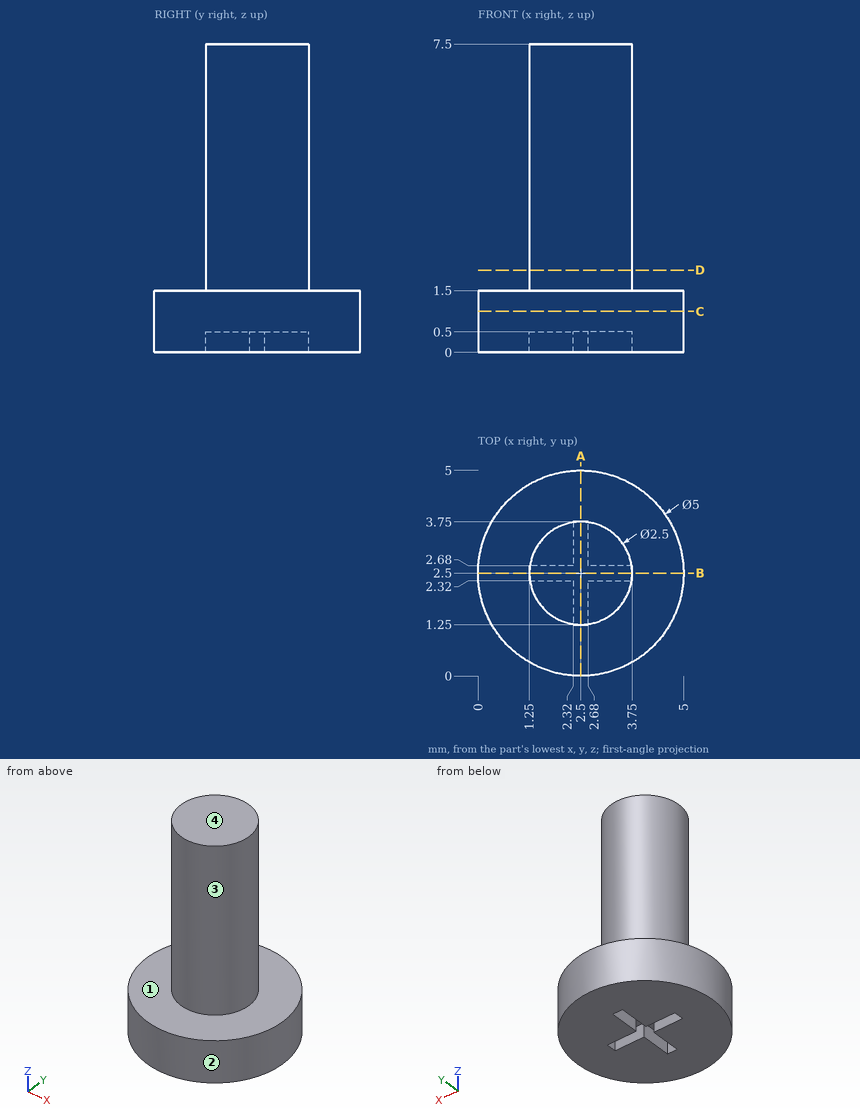
Study the drawing (mm; zero at the part's minimum x, y, z) and answer. A direction names the side the tool comes from. Give positions to 0.01 mm unless a question says otherwise; leave off trailing zeros. Write each loop counter-clockwise with the first axis right and the second up, starting at its lowest first coordinate (ties: lowest second). Pieces come first, ordered by that corner, then holes. Notation, with made-up numbers: (80, 27) - (92, 27) arc R15 ccw to (92, 52) - close; hole circle Ø1 at (-16, 68). An arc over 180 degrees is marked (long way). Use a Markdown table: item, result.
1. Section D-D on z = 2 is taken. Write down the section's boundary in (x, y).
Values follow:
| item | result |
|---|---|
| outline | circle Ø2.5 at (2.5, 2.5) |
2. A tool of negligible diameter and unlimited length cuts with its end or side. For the marked faces 1 and 2, from which of +Z, -Z, +X, -X, +Y, -Y can it reach the whole face along a straight path? Write none if from no direction.
Values follow:
| item | result |
|---|---|
| face 1 | +Z |
| face 2 | +Z, -Z |
3. Each of these flat-tipped pins is pushed along its axis until it touches: P1, Ø0.6, axis at y = 1.5, z = 0, coming from the -X side; P2, Ø0.6, axis at x = 2, z = 0.5, coming from the -Y side; P3, Ø0.8, axis at x = 2.5, y = 2.5, coming from the -Z side; P4, Ø0.6, axis at y = 3, z = 0.5, coming from the +X side. Where does it stop, or does it pass through?
Values follow:
| item | result |
|---|---|
| P1 | stops at x = 0.1 |
| P2 | stops at y = 0.01 |
| P3 | stops at z = 0 |
| P4 | stops at x = 4.99 |
4. Section A-A on x = 2.5 is taken. Write down the section's boundary in (y, z), plus the area to 4 significant figures.
Values follow:
| item | result |
|---|---|
| outline | (0, 0) - (1.25, 0) - (1.25, 0.5) - (3.75, 0.5) - (3.75, 0) - (5, 0) - (5, 1.5) - (3.75, 1.5) - (3.75, 7.5) - (1.25, 7.5) - (1.25, 1.5) - (0, 1.5) - close |
| area | 21.25 mm² |
5. Section C-C on z = 1 is taken. Write down the section's boundary in (x, y).
Values follow:
| item | result |
|---|---|
| outline | circle Ø5 at (2.5, 2.5) |
6. Find the intervals of material crossed by probe 1 along Z at (x, y) = (1.7, 0.8); probe 2 along Y at (x, z) = (1.5, 2.75); probe 3 along Z at (x, y) = (1.85, 2.4), in increasing order. Write a range as from..to.
Values follow:
| item | result |
|---|---|
| probe 1 | z = 0..1.5 |
| probe 2 | y = 1.75..3.25 |
| probe 3 | z = 0.5..7.5 |
7. For a pull along X with two mould halves and no side action, classify the marked faces 3 and 4 as released by +X, released by -X, zero draft, split by the parting line, or undercut.
Values follow:
| item | result |
|---|---|
| face 3 | split by the parting line |
| face 4 | zero draft |
